Could you check a few things on this model? Use its own coordinates, in mm. Face numbers are marked on the shaded views. A direction names the side the tool comes from. Round coordinates to 2 decimals unless told otherwise and drop trailing zeros. Order: outer loops, then holes, each group sorted by start corner. A loop starts at its lowest first (then second) coordinate and runs counter-clockwise, first axis right, second up.
```python
from build123d import *

# Parameters (mm, degrees)
SKETCH117_W     = 15
SKETCH117_H     = 44
SKETCH117_W_2   = 7
SKETCH117_H_2   = 30
PAD063_DEPTH    = 120
SKETCH118_W     = 11
SKETCH118_H     = 40
POCKET044_DEPTH = 31
SKETCH119_W     = 11
SKETCH119_H     = 40
POCKET045_DEPTH = 31
CHAMFER061_SIZE = 0.5
CHAMFER062_SIZE = 0.5


with BuildPart() as part:
    # Sketch117 → Pad063 (new body)
    with BuildSketch(Plane.XY):
        Rectangle(SKETCH117_W, SKETCH117_H)
        Rectangle(SKETCH117_W_2, SKETCH117_H_2, mode=Mode.SUBTRACT)
    extrude(amount=PAD063_DEPTH)

    # Sketch118 (on Face9 of Pad063) → Pocket044 (cut)
    with BuildSketch(Plane(origin=(0, 0, 0), x_dir=(1, 0, 0), z_dir=(0, 0, -1))):
        Rectangle(SKETCH118_W, SKETCH118_H)
    extrude(amount=-POCKET044_DEPTH, mode=Mode.SUBTRACT)

    # Sketch119 (on Face5 of Pocket044) → Pocket045 (cut)
    with BuildSketch(Plane.XY.offset(120)):
        Rectangle(SKETCH119_W, SKETCH119_H)
    extrude(amount=-POCKET045_DEPTH, mode=Mode.SUBTRACT)

    # Chamfer061
    chamfer061_edges = [part.edges().sort_by_distance(p)[0] for p in [
        (7.5, -22, 60),
        (-7.5, -22, 60),
        (-7.5, 22, 60),
        (7.5, 22, 60),
    ]]
    chamfer(chamfer061_edges, length=CHAMFER061_SIZE)

    # Chamfer062
    chamfer062_edges = [part.edges().sort_by_distance(p)[0] for p in [
        (-5.5, 0, 120),
        (0, -20, 120),
        (5.5, 0, 120),
        (0, 20, 120),
        (-5.5, 0, 0),
        (5.5, 0, 0),
        (0, -20, 0),
        (0, 20, 0),
    ]]
    chamfer(chamfer062_edges, length=CHAMFER062_SIZE)


with BuildPart() as part_1:
    # Body022 placement: moved
    add(part.part.moved(Location((-106.5, -22, -126))))


solid = part_1.part
```
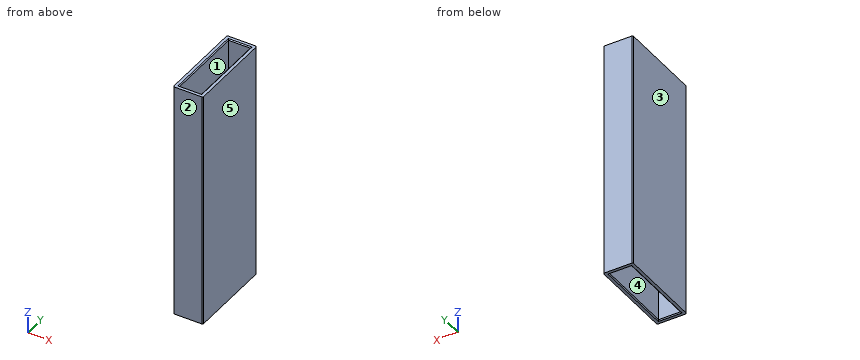
Q1. For P1, Ø2, axis at x = -104.5, y = -14, coming from the +Z side; P2, Ø3.5, axis at x = -104, y = -29.5, coming from the -Z side, each with a flat end and sliding along its axis, tell me the tip position at first contact or that it passes through.
Q2. I need wall thicknesses on L1, parallel to Y at x = -107, z = -43.5; L2, parallel to Y at x = -108.75, z = -119.5; L3, parallel to X at y = -11.5, z = -49. Which ranges of each line are inside material? Lowest first, please.
Q3. For the marked faces 4 and 5, which set-ups out of +Z, -Z, +X, -X, +Y, -Y let a thin tool reach every point of the face, with its end or its side?
Q4. Imagine slicing it at B-B, the plane z = -52. Please give me the cut outline in (x, y), then the cut area to 4 significant figures.
Q5. Imagine slicing it at A-A, the plane y = -35. Please give me the cut outline in (x, z).
Q6. Imagine slicing it at D-D, the plane z = -102. Please give me the cut outline in (x, y).
Q7. Imagine slicing it at C-C, the plane x = -107.25. Please give me the cut outline in (y, z).
Q8. We'd pull the mould along X, two halves only. Please class the marked faces 1, 2 and 3: released by +X, released by -X, zero draft, split by the parting line, or undercut.
Filled in:
1. P1: passes through
1. P2: stops at z = -95
2. L1: y = -44 to -37, -7 to 0
2. L2: y = -44 to -42, -2 to 0
2. L3: x = -114 to -110, -103 to -99
3. face 4: -Z
3. face 5: +Z, -Z, +X, +Y, -Y
4. outline: (-114, -43.5) - (-113.5, -44) - (-99.5, -44) - (-99, -43.5) - (-99, -0.5) - (-99.5, 0) - (-113.5, 0) - (-114, -0.5) - close; hole (-110, -37) - (-103, -37) - (-103, -7) - (-110, -7) - close
4. area: 449.5 mm2
5. outline: (-114, -126) - (-112.5, -126) - (-112, -125.5) - (-112, -95) - (-110, -95) - (-110, -37) - (-112, -37) - (-112, -6.5) - (-112.5, -6) - (-114, -6) - close; (-103, -95) - (-101, -95) - (-101, -125.5) - (-100.5, -126) - (-99, -126) - (-99, -6) - (-100.5, -6) - (-101, -6.5) - (-101, -37) - (-103, -37) - close
6. outline: (-114, -43.5) - (-113.5, -44) - (-99.5, -44) - (-99, -43.5) - (-99, -0.5) - (-99.5, 0) - (-113.5, 0) - (-114, -0.5) - close; hole (-112, -42) - (-101, -42) - (-101, -2) - (-112, -2) - close
7. outline: (-44, -126) - (-42.5, -126) - (-42, -125.5) - (-42, -95) - (-37, -95) - (-37, -37) - (-42, -37) - (-42, -6.5) - (-42.5, -6) - (-44, -6) - close; (-7, -95) - (-2, -95) - (-2, -125.5) - (-1.5, -126) - (0, -126) - (0, -6) - (-1.5, -6) - (-2, -6.5) - (-2, -37) - (-7, -37) - close
8. face 1: undercut
8. face 2: zero draft
8. face 3: released by -X
